Build history of the part. All positions in model axes, mm. A direction names the side the tool comes from. Round coordinates to 2 decimals unless told otherwise and drop trailing zeros. Loops run counter-clockwise (first coordinate to the right, second up) from the corner with the lowest first, then second, coordinate; pieces in that order, holes last. Notation, with made-up numbers: (72, 12.25) -> (93, 12.25) arc R32 cw to (93, 38.25) -> close; hole circle Ø1 at (29.5, -14.5). An arc over 180 degrees is marked (long way). Put each result on its own line as item: value. Start each with the question number.
Item 1: Cut at D-D, the plane y = 93.5. List the corners of the cut face in (x, z).
Item 2: Cut at B-B, the plane z = 2.5. List the corners of the cut face in (x, y), plus the area to 3 significant figures.
Item 3: Pull direction Z, two halves, no side cores. Call faces 4 (the flat face through (-2, 18.77, -2)), 5 (the flat face through (2, 8.8, 2)), 6 (the flat face through (0, 56, 4.25)): +Z half, -Z half, draft (parallel to the pull), parting line (faces both ways), or undercut.
Item 4: Flat gauge pin, fed straight in: pin 1 Ø0.8 at (x, y) = (2.5, 91) entering from +Z. Where does the tip first touch, or does it go through?
Item 5: Tool access for faces 1 (the flat face through (0, 0, 0)), 2 (the flat face through (-2, 23, -0.75)), 3 (the flat face through (2, 18.3, 2)): list every direction of +Z, -Z, +X, -X, +Y, -Y with a clear straight run to the whole face (end or side of a thin tool).
Item 6: Cut at C-C, the plane x = -2.75. List the corners of the cut face in (y, z).
Item 7: Drill centre lines: probe 1 along Y at (x, z) = (3, 0.25); probe 2 along Y at (x, z) = (-3.5, -1); probe 3 along Z at (x, y) = (0.25, 26). Where is each one in solid material? Low to high. Write a range as [from, to].
Item 8: Cut at A-A, the plane x = 2. List the corners of the cut face in (y, z), plus the area to 3 significant figures.
```python
from build123d import *

# Parameters (mm, degrees)
SKETCH1_W           = 8.5
SKETCH1_H           = 8.5
BOSS_EXTRUDE1_DEPTH = 113.5
SKETCH2_W           = 2.5
SKETCH2_H           = 9.5
CUT_EXTRUDE1_DEPTH  = 5
SKETCH3_W           = 2.5
SKETCH3_H           = 9.5
CUT_EXTRUDE2_DEPTH  = 5


with BuildPart() as part:
    # Sketch1 → Boss-Extrude1 (new body)
    with BuildSketch(Plane(origin=(0, 0, 0), x_dir=(1, 0, 0), z_dir=(0, 1, 0))):
        Rectangle(SKETCH1_W, SKETCH1_H)
    extrude(amount=BOSS_EXTRUDE1_DEPTH)

    # Sketch2 → Cut-Extrude1 (cut)
    with BuildSketch(Plane.XY.offset(4.25)):
        with Locations((2, 13.55)):
            Rectangle(SKETCH2_W, SKETCH2_H)
        with Locations((2, 89.98)):
            Rectangle(SKETCH2_W, SKETCH2_H)
    extrude(amount=-CUT_EXTRUDE1_DEPTH, mode=Mode.SUBTRACT)

    # Sketch3 → Cut-Extrude2 (cut)
    with BuildSketch(Plane.ZY.offset(4.25)):
        with Locations((-2, 99.95)):
            Rectangle(SKETCH3_W, SKETCH3_H)
        with Locations((-2, 23.52)):
            Rectangle(SKETCH3_W, SKETCH3_H)
    extrude(amount=-CUT_EXTRUDE2_DEPTH, mode=Mode.SUBTRACT)


solid = part.part
```
Reply:
1. outline: (-4.25, -4.25) -> (4.25, -4.25) -> (4.25, 4.25) -> (3.25, 4.25) -> (3.25, -0.75) -> (0.75, -0.75) -> (0.75, 4.25) -> (-4.25, 4.25) -> close
2. outline: (-4.25, 0) -> (4.25, 0) -> (4.25, 113.5) -> (-4.25, 113.5) -> close; hole (0.75, 8.8) -> (3.25, 8.8) -> (3.25, 18.3) -> (0.75, 18.3) -> close; hole (0.75, 85.23) -> (3.25, 85.23) -> (3.25, 94.73) -> (0.75, 94.73) -> close
2. area: 917 mm^2
3. face 4: undercut
3. face 5: draft
3. face 6: +Z half
4. pin 1: stops at z = -0.75
5. face 1: +Z, -Z, +X, -X, -Y
5. face 2: -X
5. face 3: +Z
6. outline: (0, -4.25) -> (113.5, -4.25) -> (113.5, 4.25) -> (0, 4.25) -> close; hole (18.77, -3.25) -> (28.27, -3.25) -> (28.27, -0.75) -> (18.77, -0.75) -> close; hole (95.2, -3.25) -> (104.7, -3.25) -> (104.7, -0.75) -> (95.2, -0.75) -> close
7. probe 1: y = [0, 8.8], [18.3, 85.23], [94.73, 113.5]
7. probe 2: y = [0, 18.77], [28.27, 95.2], [104.7, 113.5]
7. probe 3: z = [-4.25, -3.25], [-0.75, 4.25]
8. outline: (0, -4.25) -> (113.5, -4.25) -> (113.5, 4.25) -> (94.73, 4.25) -> (94.73, -0.75) -> (85.23, -0.75) -> (85.23, 4.25) -> (18.3, 4.25) -> (18.3, -0.75) -> (8.8, -0.75) -> (8.8, 4.25) -> (0, 4.25) -> close
8. area: 870 mm^2
